```python
from build123d import *

# Parameters (mm, degrees)
SKETCH_R     = 3
PAD_DEPTH    = 3
SKETCH001_R  = 1
POCKET_DEPTH = 3.001
FILLET_R     = 3
CHAMFER_SIZE = 0.5


with BuildPart() as part:
    # Sketch → Pad (new body)
    with BuildSketch(Plane.XY):
        Polygon((-35, 29.15), (-35, 1.5), (35, 1.5), (35, 29.15), (50, 29.15), (50, -1.5), (-50, -1.5), (-50, 29.15), align=None)
        with Locations((-44.075, 18.17)):
            Circle(SKETCH_R, mode=Mode.SUBTRACT)
        with Locations((44.075, 18.17)):
            Circle(SKETCH_R, mode=Mode.SUBTRACT)
    extrude(amount=PAD_DEPTH)

    # Sketch001 → Pocket (cut, through all)
    with BuildSketch(Plane.XY.offset(3)):
        with Locations((-35, 1.5)):
            Circle(SKETCH001_R)
        with Locations((35, 1.5)):
            Circle(SKETCH001_R)
    extrude(amount=-POCKET_DEPTH, mode=Mode.SUBTRACT)

    # Fillet
    fillet_edges = [part.edges().sort_by_distance(p)[0] for p in [
        (-35, 29.15, 1.5),
        (35, 29.15, 1.5),
    ]]
    fillet(fillet_edges, radius=FILLET_R)

    # Chamfer
    chamfer_edges = [part.edges().sort_by_distance(p)[0] for p in [
        (0, 1.5, 0),
        (-35, 14.325, 0),
        (35, 14.325, 0),
        (-35.87868, 28.27132, 0),
        (35.87868, 28.27132, 0),
        (-47.075, 18.17, 0),
        (41.075, 18.17, 0),
    ]]
    chamfer(chamfer_edges, length=CHAMFER_SIZE)


solid = part.part
```
Geometry check sheet. Reference: the model listing, model coordinates, mm. A direction names the side the tool comes from. Round coordinates to 2 decimals unless told otherwise and drop trailing zeros. Order: outer loops, then holes, each group sorted by start corner. A loop starts at its lowest first (then second) coordinate and runs counter-clockwise, first axis right, second up. Notation, with made-up numbers: M 43.25,26.5 L 74.25,26.5 A23 cw 74.25,46.5 Z; hole C 86.25,-25.75 d4. An arc over 180 degrees is marked long. Answer as CSV lines item,"result".
1) Sectioned sample at B-B on z = 2. Record the cut outline in (x, y) (3 decimals).
Entries:
outline,"M -50,-1.5 L 50,-1.5 L 50,29.15 L 38,29.15 A3 ccw 35,26.15 L 35,2.5 A1 cw long 34,1.5 L -34,1.5 A1 cw long -35,2.5 L -35,26.15 A3 ccw -38,29.15 L -50,29.15 Z; hole C -44.075,18.17 d6; hole C 44.075,18.17 d6"
2) Sectioned sample at D-D on x = 20.5. Record the cut outline in (y, z).
Entries:
outline,"M -1.5,0 L 1,0 L 1.5,0.5 L 1.5,3 L -1.5,3 Z"
3) Thickness scan on probe 1 along X at (y, z) = (18, 2.45); probe 2 along X at (y, z) = (24.5, 2.6); probe 3 along X at (y, z) = (16, 1). Record the ranges inside material, lowest first. Write a range as [from, to].
Entries:
probe 1,"[-50, -47.07], [-41.08, -35], [35, 41.08], [47.07, 50]"
probe 2,"[-50, -35], [35, 50]"
probe 3,"[-50, -46.15], [-42, -35], [35, 42], [46.15, 50]"
4) Sectioned sample at A-A on y = 18.17. Record the cut outline in (x, z) (3 decimals).
Entries:
outline,"M -50,0 L -47.575,0 L -47.075,0.5 L -47.075,3 L -50,3 Z; M -41.075,0.5 L -40.575,0 L -35.5,0 L -35,0.5 L -35,3 L -41.075,3 Z; M 35,0.5 L 35.5,0 L 40.575,0 L 41.075,0.5 L 41.075,3 L 35,3 Z; M 47.075,0.5 L 47.575,0 L 50,0 L 50,3 L 47.075,3 Z"
5) Gauge pin test, flat ends, axial feed: pin 1 Ø3 at (x, y) = (35, 1.5) entering from -Z; pin 2 Ø1 at (x, z) = (14.5, 1.5) entering from +Y. Record the tip position at first contact, or that the pin passes through.
Entries:
pin 1,"z = 0"
pin 2,"y = 1.5"
6) Tool access check on faces 4 (the face through (0, 1.5, 2)), 5 (the face through (36.111, 27.998, 0.142)), 6 (the face through (50, 14, 1)). Record the directions out of +Z, -Z, +X, -X, +Y, -Y that give a thin tool (end or side, any length) a straight path to the whole face; none if there is none.
Entries:
face 4,"+Z, -Z, +Y"
face 5,"-Z, +Y"
face 6,"+Z, -Z, +X, +Y, -Y"
7) Sectioned sample at C-C on y = 5. Record the cut outline in (x, z), and give its area (4 significant figures).
Entries:
outline,"M -50,0 L -35.5,0 L -35,0.5 L -35,3 L -50,3 Z; M 35,0.5 L 35.5,0 L 50,0 L 50,3 L 35,3 Z"
area,"89.75 mm2"
8) Mould release check, pull along Y, two halves, no side actions. Record for faces 1 (the face through (-35.86, 28.25, 1.77)), 2 (the face through (35, 14, 2)), 3 (the face through (35.683, 0.77, 1.521)): +Y half, -Y half, draft (parallel to the pull), parting line (faces both ways), or undercut.
Entries:
face 1,"+Y half"
face 2,"draft"
face 3,"undercut"
